```python
from build123d import *

# Parameters (mm, degrees)
ESBO_O1_R                = 85
RESSALTO_EXTRUS_O1_DEPTH = 6


with BuildPart() as part:
    # Esboço1 → Ressalto-extrusão1 (new body)
    with BuildSketch(Plane(origin=(0, 0, 0), x_dir=(1, 0, 0), z_dir=(0, 1, 0))):
        with Locations(Location((0, 0, 0), (0, 0, 270))):
            Circle(ESBO_O1_R)
        with BuildLine():
            Line((-54.083269132, -10), (-10, -10))
            Line((-10, -10), (-10, -54.083269132))
            ThreePointArc((-10, -54.083269132), (-38.890872965, -38.890872965), (-54.083269132, -10))
        make_face(mode=Mode.SUBTRACT)
        with BuildLine():
            Line((10, -54.083269132), (10, -10))
            Line((10, -10), (54.083269132, -10))
            ThreePointArc((54.083269132, -10), (38.890872965, -38.890872965), (10, -54.083269132))
        make_face(mode=Mode.SUBTRACT)
        with BuildLine():
            Line((54.083269132, 10), (10, 10))
            Line((10, 10), (10, 54.083269132))
            ThreePointArc((10, 54.083269132), (38.890872965, 38.890872965), (54.083269132, 10))
        make_face(mode=Mode.SUBTRACT)
        with BuildLine():
            Line((-10, 54.083269132), (-10, 10))
            Line((-10, 10), (-54.083269132, 10))
            ThreePointArc((-54.083269132, 10), (-38.890872965, 38.890872965), (-10, 54.083269132))
        make_face(mode=Mode.SUBTRACT)
    extrude(amount=RESSALTO_EXTRUS_O1_DEPTH)


solid = part.part
```
Part model, mm, in its own coordinate system. A direction names the side the tool comes from. Round coordinates to 2 decimals unless told otherwise and drop trailing zeros. Write each loop counter-clockwise with the first axis right and the second up, starting at its lowest first coordinate (ties: lowest second). Pieces come first, ordered by that corner, then holes.
Item 1: Drop flat-ended pins along their axis: pin 1 Ø3 at (x, y) = (10, 4) entering from +Z; pin 2 Ø1.8 at (x, y) = (-37, 3.5) entering from +Z; pin 3 Ø3 at (x, y) = (22.5, 2.5) entering from +Z. Give the stop position or say it passes through.
Results:
pin 1: stops at z = 84.57
pin 2: stops at z = 76.95
pin 3: stops at z = 82.37
Item 2: Cut at B-B, the plane z = -51.5. Give the cut face in (x, y), plus the area to 3 significant figures.
Results:
outline: (-67.62, 0) - (-19.31, 0) - (-19.31, 6) - (-67.62, 6) - close; (-10, 0) - (10, 0) - (10, 6) - (-10, 6) - close; (19.31, 0) - (67.62, 0) - (67.62, 6) - (19.31, 6) - close
area: 700 mm2
Item 3: Cut at A-A, the plane y = 4. Give the cut face in (x, z).
Results:
outline: circle Ø170 at (0, 0); hole (-54.08, -10) arc R55 ccw to (-10, -54.08) - (-10, -10) - close; hole (-54.08, 10) - (-10, 10) - (-10, 54.08) arc R55 ccw to start; hole (10, -54.08) arc R55 ccw to (54.08, -10) - (10, -10) - close; hole (10, 10) - (54.08, 10) arc R55 ccw to (10, 54.08) - close
Item 4: Which spindle directions (+Z, -Z, +X, -X, +Y, -Y) get a long thin tool onto all of the face, cutting with end or side? Do faces 5 (the flat face through (1, 6, -1)), 6 (the flat face through (32, 3, -10)). Say none if no direction does.
Results:
face 5: +Z, -Z, +X, -X, +Y
face 6: +Y, -Y
Item 5: Probe L1, parallel to X at y = 5.45, z = 13.5; L2, parallel to X at y = 5.4, z = -29.5; L3, parallel to Z at x = -14.5, y = 3.35. List the from-to ranges inside material, lowest first.
Results:
L1: x = -83.92 to -53.32, -10 to 10, 53.32 to 83.92
L2: x = -79.72 to -46.42, -10 to 10, 46.42 to 79.72
L3: z = -83.75 to -53.05, -10 to 10, 53.05 to 83.75
Item 6: Two-plate mould, pull along X, no slides. Class faces 1 (the cylindrical face through (-51.721, 2.958, -67.453)), 2 (the cylindrical face through (39.22, 2.96, 38.56)), 3 (the flat face through (1, 0, -1)), 4 (the cylindrical face through (38.56, 2.96, -39.22)): +X half, -X half, draft (parallel to the pull), parting line (faces both ways), or undercut.
Results:
face 1: parting line
face 2: undercut
face 3: draft
face 4: undercut
Item 7: Cut at C-C, the plane x = -46.5. Give the cut face in (y, z), plus the area to 3 significant figures.
Results:
outline: (0, -71.15) - (6, -71.15) - (6, -29.37) - (0, -29.37) - close; (0, -10) - (6, -10) - (6, 10) - (0, 10) - close; (0, 29.37) - (6, 29.37) - (6, 71.15) - (0, 71.15) - close
area: 621 mm2
